```python
from build123d import *

# Parameters (mm, degrees)
BOSS_EXTRUDE1_DEPTH = 14.2875
SKETCH2_R           = 6.33095
CUT_EXTRUDE1_DEPTH  = 12.90625


with BuildPart() as part:
    # Sketch1 → Boss-Extrude1 (new body, symmetric)
    with BuildSketch(Plane(origin=(0, 0, 0), x_dir=(0, 0, -1), z_dir=(1, 0, 0))):
        Polygon((7.9375, 11.90625), (-7.9375, 11.90625), (-7.9375, 7.9375), (-14.2875, 7.9375), (-14.2875, 0), (14.2875, 0), (14.2875, 7.9375), (7.9375, 7.9375), align=None)
    extrude(amount=BOSS_EXTRUDE1_DEPTH, both=True)

    # Sketch2 → Cut-Extrude1 (cut, through all)
    with BuildSketch(Plane(origin=(0, 11.90625, 0), x_dir=(1, 0, 0), z_dir=(0, 1, 0))):
        Circle(SKETCH2_R)
    extrude(amount=-CUT_EXTRUDE1_DEPTH, mode=Mode.SUBTRACT)


solid = part.part
```
Can you work these out from the model? Positions are in its coordinate system, mm. A direction names the side the tool comes from. Round coordinates to 2 decimals unless told otherwise and drop trailing zeros. Order: outer loops, then holes, each group sorted by start corner. A loop starts at its lowest first (then second) coordinate and runs counter-clockwise, first axis right, second up.
(1) If I drill on L1, parallel to X at y = 6.25, z = 0; L2, parallel to Z at x = 0, y = 9, over which ranges is the centre line in solid material (lowest first)?
Results are:
L1: x = -14.29 to -6.33, 6.33 to 14.29
L2: z = -7.94 to -6.33, 6.33 to 7.94
(2) I'm going to push flat-ended pins straight in: pin 1 (4.5 mm diameter, centred on x = 4.5, y = 10.5, fed in from +Z); pin 2 (2 mm diameter, centred on x = 2.5, y = 10.5, fed in from -Z); pin 3 (5 mm diameter, centred on x = -3, z = -12.5, fed in from +Y); pin 4 (5 mm diameter, centred on x = 10, z = -3, fed in from -Y). Where does each tip first touch, or does it pass through?
Results are:
pin 1: stops at z = 7.94
pin 2: stops at z = -7.94
pin 3: stops at y = 7.94
pin 4: stops at y = 0
(3) If we section it at D-D (x = 5): Please give me the cut outline in (y, z), plus the area to 3 significant figures.
Results are:
outline: (0, -14.29) - (7.94, -14.29) - (7.94, -7.94) - (11.91, -7.94) - (11.91, -3.88) - (0, -3.88) - close; (0, 3.88) - (11.91, 3.88) - (11.91, 7.94) - (7.94, 7.94) - (7.94, 14.29) - (0, 14.29) - close
area: 197 mm2
(4) If we section it at B-B (x = 0): Please give me the cut outline in (y, z), plus the area to 3 significant figures.
Results are:
outline: (0, -14.29) - (7.94, -14.29) - (7.94, -7.94) - (11.91, -7.94) - (11.91, -6.33) - (0, -6.33) - close; (0, 6.33) - (11.91, 6.33) - (11.91, 7.94) - (7.94, 7.94) - (7.94, 14.29) - (0, 14.29) - close
area: 139 mm2
(5) We'd pull the mould along X, two halves only. Please class faces 4 (the face through (0, 4, 14.288)), 5 (the face through (-6.325, 6.036, -0.278)), 6 (the face through (14.288, 5, 0)), 7 (the face through (-14.288, 5, 0)): +X half, -X half, draft (parallel to the pull), parting line (faces both ways), or undercut.
Results are:
face 4: draft
face 5: undercut
face 6: +X half
face 7: -X half
(6) If we section it at C-C (x = -9): Please give me the cut outline in (y, z), plus the area to 3 significant figures.
Results are:
outline: (0, -14.29) - (7.94, -14.29) - (7.94, -7.94) - (11.91, -7.94) - (11.91, 7.94) - (7.94, 7.94) - (7.94, 14.29) - (0, 14.29) - close
area: 290 mm2
(7) On a 3-axis mill with a long thin cutter (end or side, diameter ignored), from which of +Z, -Z, +X, -X, +Y, -Y can I reach the whole of each face in a straight line? I mean faces 1 (the face through (0, 10, 7.938)), 2 (the face through (7, 0, 0)), 3 (the face through (0, 10, -7.938)). Say none if no direction works.
Results are:
face 1: +Z, +X, -X, +Y
face 2: +Z, -Z, +X, -X, -Y
face 3: -Z, +X, -X, +Y
(8) If we section it at A-A (z = 0): Please give me the cut outline in (x, y), plus the area to 3 significant figures.
Results are:
outline: (-14.29, 0) - (-6.33, 0) - (-6.33, 11.91) - (-14.29, 11.91) - close; (6.33, 0) - (14.29, 0) - (14.29, 11.91) - (6.33, 11.91) - close
area: 189 mm2
